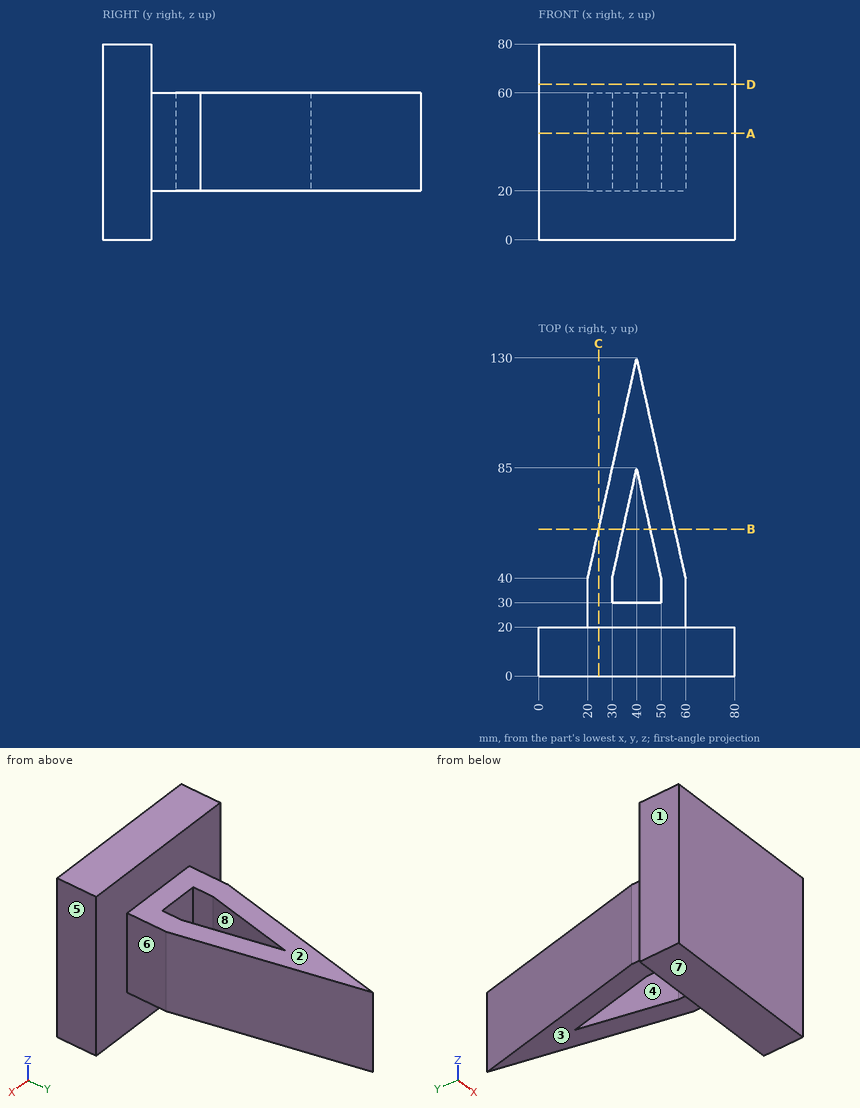
Geometry check sheet. Reference: drawing and pictorial views, mm from the part's lowest x, y, z. A direction names the side the tool comes from. Give positions to 0.01 mm unless a question says otherwise; leave off trailing zeros. Order: outer loops, then holes, each group sorted by start corner. A loop starts at its lowest first (then second) coordinate and runs counter-clockwise, first axis right, second up. Notation, with made-up numbers: M 48.25,-26.5 L 76.25,-26.5 A24 cw 76.25,4.5 Z; hole C -34.5,18 d11. An arc over 180 degrees is marked long. Answer as a JSON object with one key per item and string values. Group by question number.
1) Cross-section at A-A (z = 43.5). Enter the section's corners in (x, y), then the cut area to 3 significant figures.
2) Scan lines: line 1 along Y through (x, z) = (35.5, 63); line 2 along Z through (x, y) = (52, 71); line 3 along X through (y, z) = (38, 20.5). Record each from-to range of solid material in increasing order. Write a range as [from, to].
3) Mould release check, pull along X, two halves, no side actions. Record for the marked faces 6, 7 and 8: released by +X, released by -X, zero draft, split by the parting line, or undercut.
4) Cross-section at B-B (y = 60). Enter the section's corners in (x, z).
5) Depth check by flat-ended pin: pin 1 Ø6 at (y, z) = (115.5, 48.5) entering from -X; pin 2 Ø10 at (y, z) = (26, 39.5) entering from -X; pin 3 Ø8 at (y, z) = (37.5, 39.5) entering from +X. Enter the tip coordinate at first touch or a pass-through.
6) Cross-section at D-D (z = 63.5). Enter the section's corners in (x, y).
7) Cross-section at C-C (x = 24.5). Enter the section's corners in (y, z).
8) Access from +Z, -Z, +X, -X, +Y, -Y to the whole of each face (thin tool, end or side, straight path). Record for the marked faces 1, 2, 3, 4 and 5.
Result sheet:
{
 "1": {"outline": "M 0,0 L 80,0 L 80,20 L 60,20 L 60,40 L 40,130 L 20,40 L 20,20 L 0,20 Z; hole M 30,30 L 50,30 L 50,40 L 40,85 L 30,40 Z", "area": "3,550 mm2"},
 "2": {"line 1": "y = [0, 20]", "line 2": "z = [20, 60]", "line 3": "x = [20, 30], [50, 60]"},
 "3": {"face 6": "released by +X", "face 7": "zero draft", "face 8": "undercut"},
 "4": {"outline": "M 24.44,20 L 34.44,20 L 34.44,60 L 24.44,60 Z; M 45.56,20 L 55.56,20 L 55.56,60 L 45.56,60 Z"},
 "5": {"pin 1": "stops at x = 36.11", "pin 2": "stops at x = 20", "pin 3": "stops at x = 60"},
 "6": {"outline": "M 0,0 L 80,0 L 80,20 L 0,20 Z"},
 "7": {"outline": "M 0,0 L 20,0 L 20,20 L 60.25,20 L 60.25,60 L 20,60 L 20,80 L 0,80 Z"},
 "8": {"face 1": "+Z, -Z, -X, +Y, -Y", "face 2": "+Z, +X, -X, +Y", "face 3": "-Z, +X, -X, +Y", "face 4": "+Z, -Z", "face 5": "+Z, -Z, +X, +Y, -Y"}
}
